Build history of the part. All positions in model axes, mm. A direction names the side the tool comes from. Give positions to 0.01 mm unless a question says otherwise; leave off trailing zeros. Loops run counter-clockwise (first coordinate to the right, second up) from the corner with the lowest first, then second, coordinate; pieces in that order, holes last. Notation, with made-up numbers: M 78,19 L 91,19 A18 ccw 91,29 Z; hole C -20.5,28.5 d9. An arc over 180 degrees is marked long. Answer as a JSON object with one key per item and string values. Group by question number.
1. Slice it at C-C (z = -14). List the corners of the cut face in (x, y), then the cut area to 3 significant figures.
2. Slice it at D-D (z = -63.5). List the corners of the cut face in (x, y).
3. Slice it at A-A (y = 10). List the corners of the cut face in (x, z).
4. Mould opens along Z. For faces 5 (the face through (25, 24, -84.686)), 6 (the face through (7, 3, 15)), 7 (the face through (20.549, 5.535, 27.849)), 8 (the face through (20, 45, 34)) say: released by +Z, released by -Z, zero draft, split by the parting line, or undercut.
5. Drill centre lines: line 1 along Z through (x, y) = (23, 18); line 2 along Y through (x, z) = (-4.5, 1); line 3 along X through (y, z) = (24, -8). Where is each one in solid material? Low to high. Write a range as [from, to].
6. 3-axis set-ups, long thin cutter, end or side, ignore diameter. For faces 1 (the face through (25, 44.5, 36)), 2 (the face through (23.488, 24, -47)), 3 (the face through (21.52, 0.25, -3.29)), 4 (the face through (25, 46, -15.886)): which of +Z, -Z, +X, -X, +Y, -Y reach the whole face in a straight line?
7. Drop flat-ended pins along their axis: pin 1 Ø3.5 at (x, y) = (25, 47) entering from +Z; pin 2 Ø2 at (x, z) = (3.5, 27) entering from +Y; pin 3 Ø0.7 at (x, z) = (25, -11) entering from +Y; pin 4 Ø3 at (x, z) = (22.54, 36.36) entering from +Y. Give the stop position or say it passes through.
8. Slice it at B-B (x = 14). List the corners of the cut face in (y, z), then the cut area to 3 significant figures.
from build123d import *

# Parameters (mm, degrees)
SKETCH1_R           = 1.6
BOSS_EXTRUDE1_DEPTH = 3
SKETCH2_W           = 10
SKETCH2_H           = 10
BOSS_EXTRUDE2_DEPTH = 42
CHAMFER1_SIZE       = 5
SKETCH3_R           = 2.1
CUT_EXTRUDE1_DEPTH  = 52
SKETCH4_R           = 2.65
CUT_EXTRUDE2_DEPTH  = 0.5
SKETCH5_W           = 3
SKETCH5_H           = 43
BOSS_EXTRUDE3_DEPTH = 75
SKETCH6_W           = 3
SKETCH6_H           = 72.7
BOSS_EXTRUDE4_DEPTH = 2
SKETCH7_W           = 3
SKETCH7_H           = 68.8
BOSS_EXTRUDE5_DEPTH = 3


with BuildPart() as part:
    # Sketch1 → Boss-Extrude1 (new body)
    with BuildSketch(Plane(origin=(0, 0, 0), x_dir=(1, 0, 0), z_dir=(0, 1, 0))):
        Polygon((-6.512396694, 9.685950413), (1.487603306, 9.685950413), (26.487603306, 9.685950413), (26.487603306, -40.314049587), (1.487603306, -40.314049587), (-6.512396694, -40.314049587), align=None)
        with Locations(Location((-1.962396694, -35.764049587, 0), (0, 0, 270))):
            Circle(SKETCH1_R, mode=Mode.SUBTRACT)
        with Locations(Location((-1.962396694, 5.135950413, 0), (0, 0, 270))):
            Circle(SKETCH1_R, mode=Mode.SUBTRACT)
    extrude(amount=BOSS_EXTRUDE1_DEPTH)

    # Sketch2 → Boss-Extrude2 (add)
    with BuildSketch(Plane(origin=(0, 3, 0), x_dir=(1, 0, 0), z_dir=(0, 1, 0))):
        with Locations((21.487603306, -35.314049587)):
            Rectangle(SKETCH2_W, SKETCH2_H)
        with Locations((21.487603306, 4.685950413)):
            Rectangle(SKETCH2_W, SKETCH2_H)
    extrude(amount=BOSS_EXTRUDE2_DEPTH)

    # Chamfer1
    chamfer1_edges = [part.edges().sort_by_distance(p)[0] for p in [
        (21.487603306, 3, 30.314049587),
        (16.487603306, 3, 35.314049587),
        (16.487603306, 3, -4.685950413),
        (21.487603306, 3, 0.314049587),
    ]]
    chamfer(chamfer1_edges, length=CHAMFER1_SIZE)

    # Sketch3 → Cut-Extrude1 (cut)
    with BuildSketch(Plane(origin=(0, 45, 0), x_dir=(1, 0, 0), z_dir=(0, 1, 0))):
        with Locations(Location((22.537603306, -36.364049587, 0), (0, 0, 270))):
            Circle(SKETCH3_R)
        with Locations(Location((22.537603306, 5.735950413, 0), (0, 0, 270))):
            Circle(SKETCH3_R)
    extrude(amount=-CUT_EXTRUDE1_DEPTH, mode=Mode.SUBTRACT)

    # Sketch4 → Cut-Extrude2 (cut)
    with BuildSketch(Plane(origin=(0, 45, 0), x_dir=(1, 0, 0), z_dir=(0, 1, 0))):
        with Locations(Location((22.537603306, -36.364049587, 0), (0, 0, 270))):
            Circle(SKETCH4_R)
        with Locations(Location((22.537603306, 5.735950413, 0), (0, 0, 270))):
            Circle(SKETCH4_R)
    cut_extrude2 = extrude(amount=-CUT_EXTRUDE2_DEPTH, mode=Mode.SUBTRACT)

    # Mirror1: Cut-Extrude2 across plane
    add(cut_extrude2.mirror(Plane(origin=(0, 22.5, 0), x_dir=(0, 0, 1), z_dir=(0, -1, 0))), mode=Mode.SUBTRACT)

    # Sketch5 → Boss-Extrude3 (add)
    with BuildSketch(Plane(origin=(0, 0, -9.685950413), x_dir=(-1, 0, 0), z_dir=(0, 0, -1))):
        with Locations((-24.987603306, 21.5)):
            Rectangle(SKETCH5_W, SKETCH5_H)
    extrude(amount=BOSS_EXTRUDE3_DEPTH)

    # Sketch6 → Boss-Extrude4 (add)
    with BuildSketch(Plane(origin=(0, 43, 0), x_dir=(1, 0, 0), z_dir=(0, 1, 0))):
        with Locations((24.987603306, 48.335950413)):
            Rectangle(SKETCH6_W, SKETCH6_H)
    extrude(amount=BOSS_EXTRUDE4_DEPTH)

    # Sketch7 → Boss-Extrude5 (add)
    with BuildSketch(Plane(origin=(0, 45, 0), x_dir=(1, 0, 0), z_dir=(0, 1, 0))):
        with Locations((24.987603306, 50.285950413)):
            Rectangle(SKETCH7_W, SKETCH7_H)
    extrude(amount=BOSS_EXTRUDE5_DEPTH)


solid = part.part
Established:
{
 "1": {"outline": "M 23.49,0 L 26.49,0 L 26.49,45 L 23.49,45 Z", "area": "135 mm^2"},
 "2": {"outline": "M 23.49,0 L 26.49,0 L 26.49,48 L 23.49,48 Z"},
 "3": {"outline": "M 16.49,-9.69 L 23.49,-9.69 L 23.49,-84.69 L 26.49,-84.69 L 26.49,0.31 L 16.49,0.31 Z; M 16.49,30.31 L 26.49,30.31 L 26.49,40.31 L 16.49,40.31 Z; hole C 22.54,-5.74 d4.2; hole C 22.54,36.36 d4.2"},
 "4": {"face 5": "released by -Z", "face 6": "undercut", "face 7": "undercut", "face 8": "zero draft"},
 "5": {"line 1": "z = [-9.69, -7.78], [-3.69, 0.31], [30.31, 34.32], [38.41, 40.31]", "line 2": "y = [0, 3]", "line 3": "x = [16.49, 26.49]"},
 "6": {"face 1": "+Y", "face 2": "-Z, -X, +Y, -Y", "face 3": "-Y", "face 4": "+Z, +X, -X, +Y"},
 "7": {"pin 1": "stops at z = -15.89", "pin 2": "stops at y = 3", "pin 3": "stops at y = 43", "pin 4": "passes through"},
 "8": {"outline": "M 0,-9.69 L 5.51,-9.69 L 5.51,2.8 L 3,5.31 L 3,25.31 L 5.51,27.83 L 5.51,40.31 L 0,40.31 Z", "area": "219 mm^2"}
}
